Geometry check sheet. Reference: the model listing, model coordinates, mm. Face numbers are marked on the shaded views. A direction names the side the tool comes from. Give positions to 0.01 mm unless a question says otherwise; leave off trailing zeros. Order: outer loops, then holes, each group sorted by start corner. A loop starts at its lowest first (then second) coordinate and runs counter-clockwise, first axis right, second up. Notation, with made-up numbers: M 60.5,7.5 L 79.5,7.5 A17 cw 79.5,27.5 Z; hole C 24,25.25 d4. An arc over 180 degrees is marked long. Answer as a JSON object with one key per item and string values. Group by question number.
from build123d import *

# Parameters (mm, degrees)
SKETCH1_W           = 2.0955
SKETCH1_H           = 12.7
SKETCH2_W           = 21.844
SKETCH2_H           = 9.525
BOSS_EXTRUDE1_DEPTH = 12.827
FILLET4_R           = 1.27
SKETCH3_W           = 9.652
SKETCH3_H           = 3.175
CUT_EXTRUDE1_DEPTH  = 22.844
SKETCH4_R           = 1.5875
CUT_EXTRUDE2_DEPTH  = 10.525
CUT_EXTRUDE3_REACH  = 14.827
SKETCH5_R           = 1.1303
SKETCH6_W           = 4.191
SKETCH6_H           = 12.7
CUT_EXTRUDE4_DEPTH  = 10.525


with BuildPart() as part:
    # Sketch1 → Revolve1 (revolve)
    with BuildSketch(Plane(origin=(0, 0, 0), x_dir=(1, 0, 0), z_dir=(0, 1, 0))):
        with Locations((1.04775, 6.35)):
            Rectangle(SKETCH1_W, SKETCH1_H)
    revolve(axis=Axis((0, 0, -12.7), (0, 0, 1)))

    # Sketch2 → Boss-Extrude1 (add)
    with BuildSketch(Plane.XY):
        Rectangle(SKETCH2_W, SKETCH2_H)
    extrude(amount=BOSS_EXTRUDE1_DEPTH)

    # Fillet4
    fillet4_edges = [part.edges().sort_by_distance(p)[0] for p in [
        (10.922, -4.7625, 6.4135),
        (0, 4.7625, 0),
        (10.922, 4.7625, 6.4135),
        (-10.922, 0, 0),
        (-10.922, 4.7625, 6.4135),
        (0, -4.7625, 0),
        (-10.922, -4.7625, 6.4135),
        (10.922, 0, 0),
    ]]
    fillet(fillet4_edges, radius=FILLET4_R)

    # Sketch3 → Cut-Extrude1 (cut, through all)
    with BuildSketch(Plane.ZY.offset(10.922)):
        with Locations((8.001, 0)):
            Rectangle(SKETCH3_W, SKETCH3_H)
    extrude(amount=-CUT_EXTRUDE1_DEPTH, mode=Mode.SUBTRACT)

    # Sketch4 → Cut-Extrude2 (cut, through all)
    with BuildSketch(Plane(origin=(0, 4.7625, 0), x_dir=(1, 0, 0), z_dir=(0, 1, 0))):
        with Locations((-6.35, -8.0645)):
            Circle(SKETCH4_R)
        with Locations((6.35, -8.0645)):
            Circle(SKETCH4_R)
    extrude(amount=-CUT_EXTRUDE2_DEPTH, mode=Mode.SUBTRACT)

    # Sketch5 → Cut-Extrude3 (cut, up to next)
    with BuildSketch(Plane(origin=(0, 0, 0), x_dir=(-1, 0, 0), z_dir=(0, 0, -1)), mode=Mode.PRIVATE) as cut_extrude3_sk1:
        Circle(SKETCH5_R)
    cut_extrude3_tool1 = extrude(cut_extrude3_sk1.sketch, amount=-CUT_EXTRUDE3_REACH, mode=Mode.PRIVATE) & part.part
    add(cut_extrude3_tool1.solids().sort_by_distance((0, 0, 0))[0], mode=Mode.SUBTRACT)

    # Sketch6 → Cut-Extrude4 (cut, through all)
    with BuildSketch(Plane(origin=(0, 4.7625, 0), x_dir=(1, 0, 0), z_dir=(0, 1, 0))):
        with Locations((0, 6.35)):
            Rectangle(SKETCH6_W, SKETCH6_H)
    extrude(amount=-CUT_EXTRUDE4_DEPTH, mode=Mode.SUBTRACT)


solid = part.part
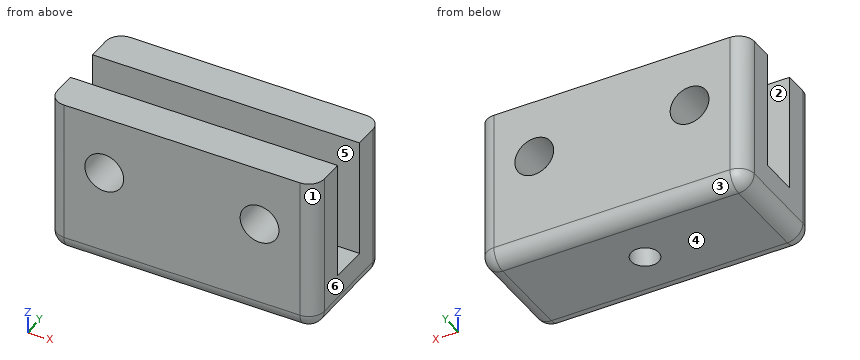
1. Cross-section at A-A (x = 0). Record the cut outline in (y, z) (1 decimal).
2. Cross-section at C-C (x = 6.35). Record the cut outline in (y, z) (1 decimal), and give its area (3 significant figures).
3. Release check for a two-part mould opening along Y. For the marked faces 1, 2, 3 and 4 record: released by +Y, released by -Y, zero draft, split by the parting line, or undercut.
4. Cross-section at D-D (z = 2). Record the cut outline in (x, y), and give its area (3 significant figures).
5. Access from +Z, -Z, +X, -X, +Y, -Y to the whole of each face (thin tool, end or side, straight path). Record for the marked faces 5 and 6.
6. Cross-section at B-B (y = 0). Record the cut outline in (x, z) (3 decimals).
7. Thickness scan on line 1 along Y through (x, z) = (4.25, 11.5); line 2 along Z through (x, y) = (-6.35, 2.3); line 3 along Y through (x, z) = (0, 2.25). Record the ranges inside material, lowest first. Write a range as [from, to].
8. Depth check by flat-ended pin: pin 1 (2.5 mm diameter, centred on x = 6.35, z = 8.06, fed in from -Y). Enter the tip coordinate at first touch or a pass-through.
Report:
{
 "1": {"outline": "M -4.8,1.3 A1.3 ccw -3.5,0 L -1.1,0 L -1.1,3.2 L -1.6,3.2 L -1.6,12.8 L -4.8,12.8 Z; M 1.1,0 L 3.5,0 A1.3 ccw 4.8,1.3 L 4.8,12.8 L 1.6,12.8 L 1.6,3.2 L 1.1,3.2 Z"},
 "2": {"outline": "M -4.8,1.3 A1.3 ccw -3.5,0 L 3.5,0 A1.3 ccw 4.8,1.3 L 4.8,6.5 L 1.6,6.5 L 1.6,3.2 L -1.6,3.2 L -1.6,6.5 L -4.8,6.5 Z; M -4.8,9.7 L -1.6,9.7 L -1.6,12.8 L -4.8,12.8 Z; M 1.6,9.7 L 4.8,9.7 L 4.8,12.8 L 1.6,12.8 Z", "area": "70.7 mm2"},
 "3": {"face 1": "released by -Y", "face 2": "undercut", "face 3": "released by +Y", "face 4": "zero draft"},
 "4": {"outline": "M -10.92,-3.49 A1.27 ccw -9.65,-4.76 L 9.65,-4.76 A1.27 ccw 10.92,-3.49 L 10.92,3.49 A1.27 ccw 9.65,4.76 L -9.65,4.76 A1.27 ccw -10.92,3.49 Z; hole C 0,0 d2.26", "area": "203 mm2"},
 "5": {"face 5": "+Z, +X, -X", "face 6": "+Z, -Z, +X, +Y, -Y"},
 "6": {"outline": "M -10.922,1.27 A1.27 ccw -9.652,0 L -1.13,0 L -1.13,3.175 L -10.922,3.175 Z; M 1.13,0 L 9.652,0 A1.27 ccw 10.922,1.27 L 10.922,3.175 L 1.13,3.175 Z"},
 "7": {"line 1": "y = [-4.76, -1.59], [1.59, 4.76]", "line 2": "z = [0, 6.48], [9.65, 12.83]", "line 3": "y = [-4.76, -1.13], [1.13, 4.76]"},
 "8": {"pin 1": "passes through"}
}
